```python
from build123d import *

# Parameters (mm, degrees)
F1_DEPTH = 6.35


with BuildPart() as f1:
    # F0 (on Top) → F1 (new body)
    with BuildSketch(Plane.XY):
        Polygon((-3.97574, 28.643733), (-3.97574, -42.725251), (14.148261, -42.725251), (14.148261, 34.510851), (29.21, 46.174749), (29.21, 77.791074), (22.86, 77.791074), (22.86, 53.314248), (17.78, 53.314248), (17.78, 77.791074), (11.43, 77.791074), (11.43, 53.450988), (6.35, 53.450988), (6.35, 77.791074), (0, 77.791074), (0, 53.450988), (-5.08, 53.450988), (-5.08, 78.309131), (-11.43, 78.309131), (-11.43, 46.174749), align=None)
    extrude(amount=F1_DEPTH)


solid = f1.part
```
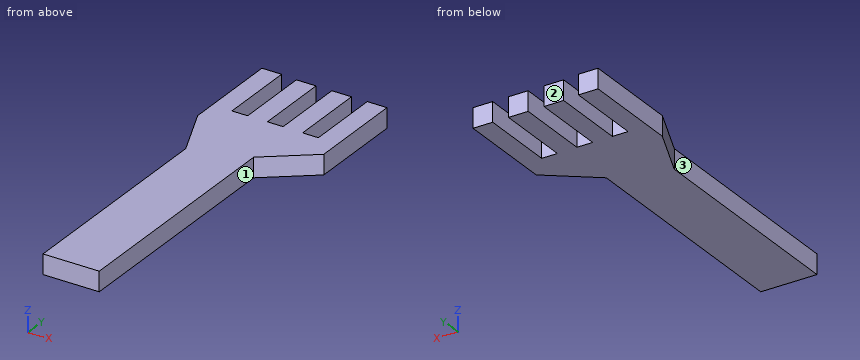
Design review of the part built by this model. Coordinates are the model's own, in mm. Face numbers are marked on the shaded views. A direction names the side the tool comes from. Coordinates: 2 decimals unless noted, no trailing zeros. Loops run counter-clockwise (first coordinate to the right, second up) from the corner with the lowest first, then second, coordinate; pieces in that order, holes last. Notation, with made-up numbers: (27.5, 40) -> (52.5, 40) arc R11 ccw to (52.5, 50) -> close; hole circle Ø8 at (56.5, 74.5). An arc over 180 degrees is marked (long way). Answer as a JSON object with one key per item and string values.
Q1. Tool access review of the marked faces 1, 2 and 3: name each direction out of +Z, -Z, +X, -X, +Y, -Y from which nothing blocks a thin tool from reaching the whole face with its end or side.
Answer block:
{"face 1": "+Z, -Z, +X, -Y", "face 2": "+Z, -Z, +X, +Y", "face 3": "+Z, -Z, -X, -Y"}
Q2. Take a section at B-B on z = 1.75. Give the boundary of the cut face in (x, y).
Answer block:
{"outline": "(-11.43, 46.17) -> (-3.98, 28.64) -> (-3.98, -42.73) -> (14.15, -42.73) -> (14.15, 34.51) -> (29.21, 46.17) -> (29.21, 77.79) -> (22.86, 77.79) -> (22.86, 53.31) -> (17.78, 53.31) -> (17.78, 77.79) -> (11.43, 77.79) -> (11.43, 53.45) -> (6.35, 53.45) -> (6.35, 77.79) -> (0, 77.79) -> (0, 53.45) -> (-5.08, 53.45) -> (-5.08, 78.31) -> (-11.43, 78.31) -> close"}
Q3. Take a section at D-D on y = 3. Give the boundary of the cut face in (x, z), plus the area to 3 significant figures.
Answer block:
{"outline": "(-3.98, 0) -> (14.15, 0) -> (14.15, 6.35) -> (-3.98, 6.35) -> close", "area": "115 mm^2"}
Q4. Take a section at C-C on x = 9. Give the boundary of the cut face in (y, z), plus the area to 3 significant figures.
Answer block:
{"outline": "(-42.73, 0) -> (53.45, 0) -> (53.45, 6.35) -> (-42.73, 6.35) -> close", "area": "611 mm^2"}
Q5. Take a section at A-A on y = 58.5. Give the boundary of the cut face in (x, z).
Answer block:
{"outline": "(-11.43, 0) -> (-5.08, 0) -> (-5.08, 6.35) -> (-11.43, 6.35) -> close; (0, 0) -> (6.35, 0) -> (6.35, 6.35) -> (0, 6.35) -> close; (11.43, 0) -> (17.78, 0) -> (17.78, 6.35) -> (11.43, 6.35) -> close; (22.86, 0) -> (29.21, 0) -> (29.21, 6.35) -> (22.86, 6.35) -> close"}
Q6. Clearance check with flat-ended pins moving along their axes: pin 1 Ø1.5 at (x, z) = (15, 4.5) entering from +Y; pin 2 Ø3 at (y, z) = (0, 4) entering from +X; pin 3 Ø1.5 at (y, z) = (36.5, 1.5) entering from +X. State where each tip first meets the part, or that it passes through.
Answer block:
{"pin 1": "stops at y = 77.79", "pin 2": "stops at x = 14.15", "pin 3": "stops at x = 17.69"}
Q7. To check wall thickness, follow L1, parallel to X at y = 55.5, z = 5.5; L2, parallel to X at y = 12, z = 2.25; L3, parallel to Y at x = 12, z = 3. State the ranges of each line that lie inside material, in increasing order.
Answer block:
{"L1": "x = -11.43 to -5.08, 0 to 6.35, 11.43 to 17.78, 22.86 to 29.21", "L2": "x = -3.98 to 14.15", "L3": "y = -42.73 to 77.79"}
